Check sheet for the modelled part. Datum: model origin and axes. Units: mm. Face numbers are marked on the shaded views. Coordinates: 2 decimals unless noted, no trailing zeros. Loops run counter-clockwise (first coordinate to the right, second up) from the corner with the lowest first, then second, coordinate; pieces in that order, holes last.
```python
from build123d import *

# Parameters (mm, degrees)
EXTRUDE_1_DEPTH          = 5
CUT_EXTRUDE_1_DEPTH      = 10.009994451
CUT_EXTRUDE_1_DEPTH_BACK = 10.009994451
SKETCH_2_OUTSIDE_W       = 15.86
SKETCH_2_OUTSIDE_H       = 15.26
CUT_EXTRUDE_3_DEPTH      = 8.698899932
SKETCH_4_R               = 0.25
CUT_EXTRUDE_4_DEPTH      = 12.980945757


with BuildPart() as part:
    # 草图1 → 拉伸-薄壁1 (new, symmetric)
    with BuildSketch(Plane(origin=(0, 0, 0), x_dir=(1, 0, 0), z_dir=(0, 1, 0))):
        with BuildLine():
            Line((5, 2), (5, 0))
            ThreePointArc((5, 0), (0, -5), (-5, 0))
            Line((-5, 0), (-5, 2))
            Line((-5, 2), (-5.3, 2))
            Line((-5.3, 2), (-5.3, 0))
            ThreePointArc((-5.3, 0), (0, -5.3), (5.3, 0))
            Line((5.3, 0), (5.3, 2))
            Line((5.3, 2), (5, 2))
        make_face()
    extrude(amount=EXTRUDE_1_DEPTH, both=True)

    # 草图2 outside → 切除-拉伸1 (cut, two sides: drawn at the far end of the back side and taken through both)
    with BuildSketch(Plane.XY.offset(-CUT_EXTRUDE_1_DEPTH_BACK)):
        Rectangle(SKETCH_2_OUTSIDE_W, SKETCH_2_OUTSIDE_H)
        with BuildLine():
            ThreePointArc((-6.091957351, 0.258709088), (0.446391065, -1.241290912), (6.98473948, 0.258709088))
            ThreePointArc((6.98473948, 0.258709088), (0.446391065, 1.758709088), (-6.091957351, 0.258709088))
        make_face(mode=Mode.SUBTRACT)
    extrude(amount=CUT_EXTRUDE_1_DEPTH + CUT_EXTRUDE_1_DEPTH_BACK, mode=Mode.SUBTRACT)

    # 草图3 → 切除-拉伸3 (cut, through all)
    with BuildSketch(Plane.XY):
        with BuildLine():
            ThreePointArc((-5.709798578, 0.166145361), (0.446391065, 1.49525914), (6.602580707, 0.166145361))
            Line((6.602580707, 0.166145361), (-5.709798578, 0.166145361))
        make_face()
        with BuildLine():
            Line((-5.709798578, 0.166145361), (6.602580707, 0.166145361))
            ThreePointArc((6.602580707, 0.166145361), (0.446391065, -1.162968417), (-5.709798578, 0.166145361))
        make_face()
    extrude(amount=CUT_EXTRUDE_3_DEPTH, mode=Mode.SUBTRACT)

    # 草图4 → 切除-拉伸4 (cut, through all)
    with BuildSketch(Plane(origin=(5.3, 0, 0), x_dir=(0, 0, -1), z_dir=(1, 0, 0))):
        with Locations((1.035921509, 0.281600465)):
            Circle(SKETCH_4_R)
    extrude(amount=-CUT_EXTRUDE_4_DEPTH, mode=Mode.SUBTRACT)


solid = part.part
```
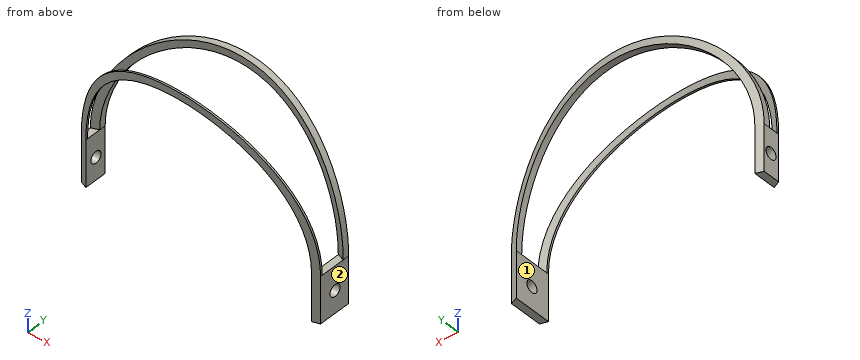
1) Section check A-A on x = 0. Enter the section's corners in (y, z), plus the area to 3 significant figures.
Answer sheet:
outline: (-1.23, 5) - (-1.16, 5) - (-1.16, 5.3) - (-1.23, 5.3) - close; (1.49, 5) - (1.75, 5) - (1.75, 5.3) - (1.49, 5.3) - close
area: 0.103 mm2
2) Section check C-C on y = 1.3. Enter the section's corners in (x, z), plus the area to 3 significant figures.
Answer sheet:
outline: (-3.23, 3.81) arc R5 cw to (-1.96, 4.6) - (-1.96, 4.92) arc R5.3 ccw to (-3.23, 4.2) - close; (2.85, 4.11) arc R5 cw to (4.13, 2.82) - (4.13, 3.32) arc R5.3 ccw to (2.85, 4.47) - close
area: 0.976 mm2
3) Mould release check, pull along X, two halves, no side actions. Record for the marked faces 1 and 2: +X half, -X half, draft (parallel to the pull), parting line (faces both ways), or undercut.
Answer sheet:
face 1: undercut
face 2: +X half
4) Scan line: line 1 (X direction, y = 0.5, z = -0.75). Record every from-to range of solid material in increasing order.
Answer sheet:
line 1: x = -5.3 to -5, 5 to 5.3
5) Section check B-B on z = 3.75. Enter the section's corners in (x, y).
Answer sheet:
outline: (-3.75, -0.64) arc R15 ccw to (-3.31, -0.76) - (-3.31, -0.68) arc R14.92 cw to (-3.75, -0.56) - close; (-3.75, 0.89) arc R14.92 cw to (-3.31, 1.02) - (-3.31, 1.28) arc R15 ccw to (-3.75, 1.16) - close; (3.31, -0.97) arc R15 ccw to (3.75, -0.87) - (3.75, -0.79) arc R14.92 cw to (3.31, -0.89) - close; (3.31, 1.22) arc R14.92 cw to (3.75, 1.13) - (3.75, 1.39) arc R15 ccw to (3.31, 1.48) - close
6) Depth check by flat-ended pin: pin 1 (1.5 mm diameter, centred on x = 3.5, y = 1, fed in from -Z); pin 2 (1 mm diameter, centred on y = 1, z = 3.5, fed in from +X); pin 3 (1 mm diameter, centred on x = -1.5, y = 1, fed in from +Z). Enter the tip coordinate at first touch or a pass-through.
Answer sheet:
pin 1: stops at z = 2.63
pin 2: stops at x = 4.37
pin 3: stops at z = 5.16
